from build123d import *

# Parameters (mm, degrees)
STOCK_GOUX_START         = 18.606590305
STOCK_GOUX_LIKED_1_DEPTH = 85.344287899
BOSS_EXTRUDE1_DEPTH      = 85.344288
SKETCH2_W                = 4
SKETCH2_H                = 5.500000112
CUT_EXTRUDE1_DEPTH       = 157.288398843
SKETCH3_R                = 0.6
CUT_EXTRUDE2_DEPTH       = 157.307592951
CIRPATTERN1_COUNT        = 2
CUT_EXTRUDE3_DEPTH       = 0.4


# Read off the part's stored shape, not the designer's step: Stock-Goux Liked-1
with BuildPart() as part:
    # Stock-Goux Liked-1 outline → Stock-Goux Liked-1 (new body)
    with BuildSketch(Plane.YZ.offset(STOCK_GOUX_START)):
        Polygon((-4.242640464, 151.610592485), (-3.889087062, 151.257039083), (0, 155.146126145), (3.889087062, 151.257039083), (4.242640464, 151.610592485), (0.707106624, 155.146126325), (3.181980438, 157.621000138), (0, 160.802980576), (-3.181980438, 157.621000138), (-0.707106624, 155.146126325), align=None)
    extrude(amount=STOCK_GOUX_LIKED_1_DEPTH)

    # Sketch1 → Boss-Extrude1 (add)
    with BuildSketch(Plane.ZY.offset(-18.606590305)):
        Polygon((151.257039083, 3.889087062), (147.367952022, 0), (151.257039083, -3.889087062), (155.146126145, 0), align=None)
    extrude(amount=-BOSS_EXTRUDE1_DEPTH)

    # Sketch2 → Cut-Extrude1 (cut, symmetric)
    with BuildSketch(Plane(origin=(0, 77.926616474, 77.926616474), x_dir=(1, 0, 0), z_dir=(-7.406550393246798e-15, 0.7071067811865402, 0.7071067811865549))):
        with Locations((20.606590305, -110.954877944)):
            Rectangle(SKETCH2_W, SKETCH2_H)
    cut_extrude1 = extrude(amount=CUT_EXTRUDE1_DEPTH, both=True, mode=Mode.SUBTRACT)

    # Sketch3 → Cut-Extrude2 (cut, through all)
    with BuildSketch(Plane(origin=(0, -76.512402912, 76.512402912), x_dir=(1, 0, 0), z_dir=(4.90653893338685e-15, -0.7071067811865547, 0.7071067811865404))):
        with Locations(Location((20.606590305, 106.704878157, 0), (0, 0, 270))):
            Circle(SKETCH3_R)
    cut_extrude2 = extrude(amount=-CUT_EXTRUDE2_DEPTH, mode=Mode.SUBTRACT)

    # CirPattern1: Cut-Extrude1, Cut-Extrude2 ×2 about axis
    cirpattern1_axis = Axis((61.278734255, 0, 0), (0, 0, 1))
    add([cut_extrude1.rotate(cirpattern1_axis, i * 360 / CIRPATTERN1_COUNT) for i in range(1, CIRPATTERN1_COUNT)], mode=Mode.SUBTRACT)
    add([cut_extrude2.rotate(cirpattern1_axis, i * 360 / CIRPATTERN1_COUNT) for i in range(1, CIRPATTERN1_COUNT)], mode=Mode.SUBTRACT)

    # Sketch4 → Cut-Extrude3 (cut)
    with BuildSketch(Plane(origin=(0, -73.683976011, 73.683976011), x_dir=(1, 0, 0), z_dir=(-7.520852272753644e-15, 0.7071067811865547, -0.7071067811865404))):
        Polygon((58.529858576, -104.856160255), (58.529858576, -108.763852563), (52.017038063, -105.42603205), (52.287981573, -104.933754406), (57.878576525, -107.799649839), (57.878576525, -104.856160255), align=None)
    extrude(amount=-CUT_EXTRUDE3_DEPTH, mode=Mode.SUBTRACT)


solid = part.part
Model file for the job. Use its own axes, mm. A direction names the side the tool comes from. Coordinates: 2 decimals unless noted, no trailing zeros. Write each loop counter-clockwise with the first axis right and the second up, starting at its lowest first coordinate (ties: lowest second). Pieces come first, ordered by that corner, then holes. Notation, with made-up numbers: (31, -25.5) - (56, -25.5) arc R30 cw to (56, 4.5) - close; hole circle Ø9 at (26.5, 82). An arc over 180 degrees is marked (long way). Write each question's results on one line, items separated by ' | '. Start each with the question number.
1) Mould opens along X. For faces 1 (the face through (22.607, 0, 156)), 2 (the face through (56.012, 1.86, 149.793)), 3 (the face through (101.979, 0.206, 152.819)) say: pulls with the +X half, pulls with the -X half, needs draft (parallel to the pull), parting line crosses it, or undercut.
2) Flat gauge pins, fed straight in: P1, Ø2, axis at x = 49, z = 150, coming from the -Y side; P2, Ø3.5, axis at y = -0.5, z = 155, coming from the +X side; P3, Ø5, axis at x = 34, z = 156.5, coming from the +Y side; P4, Ø1.5, axis at x = 37.5, y = 0.5, coming from the +Z side. Where does each tip first touch, or does it go through?
3) Cut at B-B (z = 159.75). Write the cut outline in (x, y).
4) Cut at C-C (z = 156.25). Write the cut outline in (x, y).
5) Probe line 1 along X through (y, z) = (1.25, 153.5); line 2 along Z through (x, y) = (55, -3); line 3 along X through (y, z) = (-3, 152.5). List the from-to ranges inside material, lowest first. Write a range as from..to.
6) 3-axis set-ups, long thin cutter, end or side, ignore diameter. For faces 4 (the face through (99.951, 0, 156)), 5 (the face through (55.044, 1.375, 149.022)), 6 (the face through (20.579, -0.206, 152.819)), 7 (the face through (58.709, 2.5, 153.354)), 8 (the face through (62.709, -2.45, 153.403)): which of +Z, -Z, +X, -X, +Y, -Y reach the whole face in a straight line?
7) Cut at A-A (x = 73.5). Write the cut outline in (y, z).
Returned:
1) face 1: pulls with the -X half | face 2: undercut | face 3: needs draft
2) P1: y = -3.63 | P2: x = 103.95 | P3: y = 3.18 | P4: z = 160.8
3) outline: (22.61, -1.05) - (99.95, -1.05) - (99.95, 1.05) - (22.61, 1.05) - close
4) outline: (22.61, -1.81) - (99.95, -1.81) - (99.95, 1.81) - (22.61, 1.81) - close
5) line 1: 18.61..99.95 | line 2: 150.37..152.85, 157.44..157.8 | line 3: 22.61..103.95
6) face 4: +Z, +X, +Y | face 5: +Y | face 6: +Z, -X, -Y | face 7: +X, -X, +Y | face 8: +X, -X, -Y
7) outline: (-4.24, 151.61) - (0, 147.37) - (4.24, 151.61) - (0.71, 155.15) - (3.18, 157.62) - (0, 160.8) - (-3.18, 157.62) - (-0.71, 155.15) - close
